Could you check a few things on this model? Use its own coordinates, in mm. Face numbers are marked on the shaded views. Give positions to 0.01 mm unless a question says otherwise; leave off trailing zeros. Loops run counter-clockwise (first coordinate to the right, second up) from the corner with the lowest first, then second, coordinate; pieces in that order, holes last. Notation, with made-up numbers: (-31, 34.25) - (-7, 34.25) arc R27 cw to (-7, 57.25) - close; hole circle Ø3 at (-35.5, 74). An arc over 180 degrees is marked (long way). Answer in a Markdown table with one row per item. Add a question column.
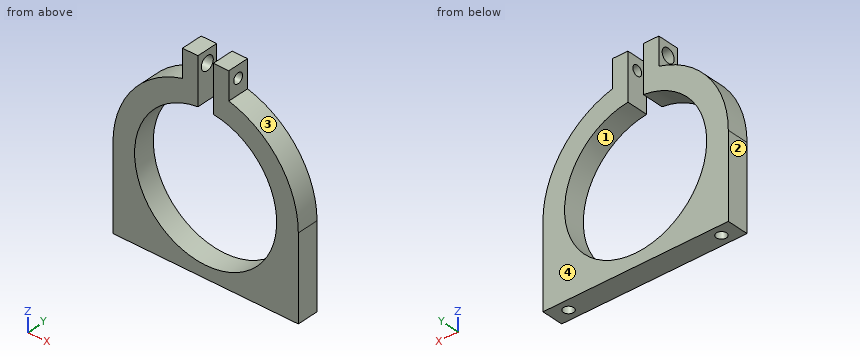
```python
from build123d import *

# Parameters (mm, degrees)
BOSS_EXTRUDE1_DEPTH   = 3.5
M4_TAPPED_HOLE2_D     = 3.3
M4_TAPPED_HOLE2_DEPTH = 9.008579979
M4_TAPPED_HOLE2_TIP   = 0.991420021
CUT_EXTRUDE1_REACH    = 55.502
SKETCH4_R             = 2.25
M4_TAPPED_HOLE1_D     = 3.3
M4_TAPPED_HOLE1_DEPTH = 9.108579979
M4_TAPPED_HOLE1_TIP   = 0.991420021


with BuildPart() as part:
    # Sketch1 → Boss-Extrude1 (new, symmetric)
    with BuildSketch(Plane(origin=(0, 0, 0), x_dir=(1, 0, 0), z_dir=(0, 1, 0))):
        with BuildLine():
            Line((-30, 0), (-30, 27))
            Line((-30, 27), (30, 27))
            Line((30, 27), (30, 0))
            ThreePointArc((30, 0), (23.717082451, -18.371173071), (7.5, -29.047375097))
            Line((7.5, -29.047375097), (7.5, -38))
            Line((7.5, -38), (2.5, -38))
            Line((2.5, -38), (2.5, -22.86372673))
            ThreePointArc((2.5, -22.86372673), (0, 23), (-2.5, -22.86372673))
            Line((-2.5, -22.86372673), (-2.5, -38))
            Line((-2.5, -38), (-7.5, -38))
            Line((-7.5, -38), (-7.5, -29.047375097))
            ThreePointArc((-7.5, -29.047375097), (-23.717082451, -18.371173071), (-30, 0))
        make_face()
    extrude(amount=BOSS_EXTRUDE1_DEPTH, both=True)

    # M4 Tapped Hole2
    with Locations(Plane(origin=(-24.75, 0, -27), x_dir=(-1, 0, 0), z_dir=(0, 0, -1))):
        with Locations((0, 0), (-49.5, 0)):
            Hole(M4_TAPPED_HOLE2_D / 2, depth=M4_TAPPED_HOLE2_DEPTH)
            with Locations((0, 0, -(M4_TAPPED_HOLE2_DEPTH + M4_TAPPED_HOLE2_TIP / 2))):  # 118° drill point
                Cone(0, M4_TAPPED_HOLE2_D / 2, M4_TAPPED_HOLE2_TIP, mode=Mode.SUBTRACT)

    # Sketch4 → Cut-Extrude1 (cut, up to next)
    with BuildSketch(Plane.ZY.offset(7.5), mode=Mode.PRIVATE) as cut_extrude1_sk1:
        with Locations((34, 0)):
            Circle(SKETCH4_R)
    cut_extrude1_tool1 = extrude(cut_extrude1_sk1.sketch, amount=-CUT_EXTRUDE1_REACH, mode=Mode.PRIVATE) & part.part
    add(cut_extrude1_tool1.solids().sort_by_distance((-7.5, 0, 34))[0], mode=Mode.SUBTRACT)

    # M4 Tapped Hole1
    with Locations(Plane(origin=(7.5, 0, 34), x_dir=(0, 0, 1), z_dir=(1, 0, 0))):
        with Locations((0, 0)):
            Hole(M4_TAPPED_HOLE1_D / 2, depth=M4_TAPPED_HOLE1_DEPTH)
            with Locations((0, 0, -(M4_TAPPED_HOLE1_DEPTH + M4_TAPPED_HOLE1_TIP / 2))):  # 118° drill point
                Cone(0, M4_TAPPED_HOLE1_D / 2, M4_TAPPED_HOLE1_TIP, mode=Mode.SUBTRACT)


solid = part.part
```
(1) I want a section at B-B on x = 21. Please give me the cut outline in (y, z), then the cut area to 3 significant figures.
(2) We'd pull the mould along X, two halves only. Please class the marked faces 1, 2, 3 and 4: pulls with the +X half, pulls with the -X half, needs draft (parallel to the pull), parting line crosses it, or undercut.
(3) Please list where these lines run through material, in increasing order: line 1 (Y direction, x = -24.75, z = -20.5); line 2 (X direction, y = 0.25, z = -24); line 3 (X direction, y = -2.75, z = 35).
(4) I want a section at A-A on z = 34. Please give me the cut outline in (x, y), then the cut area to 3 significant figures.
(5) For pin 1 Ø2 at (y, z) = (1.5, 35.5) entering from +X; pin 2 Ø3 at (y, z) = (1, 3) entering from +X; pin 3 Ø3 at (y, z) = (0, 34) entering from +X; pin 4 Ø3 at (y, z) = (1, 20.5) entering from -X, each with a flat end and sliding along its axis, tell me the tip position at first contact or that it passes through.
(6) I want a section at C-C on z = -15. Please give me the cut outline in (x, y).
Reported:
| question | item | result |
|---|---|---|
| 1 | outline | (-3.5, -27) - (3.5, -27) - (3.5, -9.38) - (-3.5, -9.38) - close; (-3.5, 9.38) - (3.5, 9.38) - (3.5, 21.42) - (-3.5, 21.42) - close |
| 1 | area | 208 mm² |
| 2 | face 1 | undercut |
| 2 | face 2 | pulls with the -X half |
| 2 | face 3 | pulls with the +X half |
| 2 | face 4 | needs draft |
| 3 | line 1 | -3.5 to -1.65, 1.65 to 3.5 |
| 3 | line 2 | -30 to -26.38, -23.12 to 23.12, 26.38 to 30 |
| 3 | line 3 | -7.5 to -2.5, 2.5 to 7.5 |
| 4 | outline | (-7.5, -3.5) - (-2.5, -3.5) - (-2.5, -2.25) - (-7.5, -2.25) - close; (-7.5, 2.25) - (-2.5, 2.25) - (-2.5, 3.5) - (-7.5, 3.5) - close; (2.5, -3.5) - (7.5, -3.5) - (7.5, -1.65) - (2.5, -1.65) - close; (2.5, 1.65) - (7.5, 1.65) - (7.5, 3.5) - (2.5, 3.5) - close |
| 4 | area | 31.0 mm² |
| 5 | pin 1 | x = 7.5 |
| 5 | pin 2 | x = 29.96 |
| 5 | pin 3 | through |
| 5 | pin 4 | x = -23.22 |
| 6 | outline | (-30, -3.5) - (-17.44, -3.5) - (-17.44, 3.5) - (-30, 3.5) - close; (17.44, -3.5) - (30, -3.5) - (30, 3.5) - (17.44, 3.5) - close |
